from build123d import *

# Parameters (mm, degrees)
BOSS_EXTRUDE1_DEPTH = 2.8
SKETCH2_W           = 22.2
SKETCH2_H           = 5
BOSS_EXTRUDE2_DEPTH = 2.8


with BuildPart() as part:
    # Sketch1 → Boss-Extrude1 (new body)
    with BuildSketch(Plane.XY):
        Polygon((-25, -13.75), (25, -13.75), (25, 13.75), (-25, 13.75), (-25, 23.75), (32.5, 23.75), (32.5, -23.75), (-25, -23.75), align=None)
    extrude(amount=BOSS_EXTRUDE1_DEPTH)

    # Sketch2 → Boss-Extrude2 (add)
    with BuildSketch(Plane(origin=(30, 0, 0), x_dir=(0, 0, -1), z_dir=(1, 0, 0))):
        with BuildLine():
            Line((-2.8, -7.5), (-2.8, 7.5))
            Line((-2.8, 7.5), (-50, 7.5))
            ThreePointArc((-50, 7.5), (-57.5, 0), (-50, -7.5))
            Line((-50, -7.5), (-2.8, -7.5))
        make_face()
        with BuildLine():
            Line((-50, -2.5), (-37.5, -2.5))
            ThreePointArc((-37.5, -2.5), (-35, 0), (-37.5, 2.5))
            Line((-37.5, 2.5), (-50, 2.5))
            ThreePointArc((-50, 2.5), (-52.5, 0), (-50, -2.5))
        make_face(mode=Mode.SUBTRACT)
        with Locations((-18.9, 0)):
            Rectangle(SKETCH2_W, SKETCH2_H, mode=Mode.SUBTRACT)
    extrude(amount=-BOSS_EXTRUDE2_DEPTH)


solid = part.part
Can you work these out from the model? Positions are in its coordinate system, mm. A direction names the side the tool comes from. Round coordinates to 2 decimals unless told otherwise and drop trailing zeros. Loops run counter-clockwise (first coordinate to the right, second up) from the corner with the lowest first, then second, coordinate; pieces in that order, holes last. Notation, with made-up numbers: (36.5, 66.25) - (62.5, 66.25) arc R7 ccw to (62.5, 76.25) - close; hole circle Ø1 at (-10.75, -18.75). An arc over 180 degrees is marked (long way). Answer in a Markdown table with one row per item. Add a question column.
Q1. I want a section at C-C on x = -16. List the corners of the cut face in (y, z) for me.
Q2. We'd pull the mould along Y, two halves only. Please class faces 6 (the flat face through (29, 0, 7.8)), 7 (the flat face through (4, 16, 0)), 8 (the cylindrical face through (29, 0, 35)), 9 (the flat face through (3, 23.75, 1)): pulls with the +Y half, pulls with the -Y half, needs draft (parallel to the pull), parting line crosses it, or undercut.
Q3. I want a section at A-A on y = 0. List the corners of the cut face in (x, z) for me.
Q4. I want a section at B-B on z = 23. List the corners of the cut face in (x, y) for me.
Q5. I want a section at D-D on z = 33.5. List the corners of the cut face in (x, y) for me.
Q6. Which directions (+Z, -Z, +X, -X, +Y, -Y) give clear straight access to the entire face, cutting with the end or side of a thin tool? Please do faces 1 (the flat face through (29, -7.5, 27)), 2 (the flat face through (25, 0, 1)), 3 (the flat face through (30, 0, 31)), 4 (the cylindrical face through (28.6, 0.1, 52.5)), 5 (the flat face through (29, 7.5, 26)).
Q7. I need wall thicknesses on L1, parallel to Y at x = 27.5, z = 40; L2, parallel to Z at x = -7.5, y = -15; L3, parallel to X at y = -3, z = 17.5. Which ranges of each line are inside material? Lowest first, please.
Q8. For pin 1 Ø0.8 at (x, z) = (29, 18) entering from -Y; pin 2 Ø7.5 at (y, z) = (2, 43.5) entering from -X; pin 3 Ø1 at (x, y) = (21, 19) entering from +Z; pin 4 Ø5 at (y, z) = (11.5, 39) entering from +X, each with a flat end and sliding along its axis, tell me the tip position at first contact or that it passes through.
A:
| question | item | result |
|---|---|---|
| 1 | outline | (-23.75, 0) - (-13.75, 0) - (-13.75, 2.8) - (-23.75, 2.8) - close; (13.75, 0) - (23.75, 0) - (23.75, 2.8) - (13.75, 2.8) - close |
| 2 | face 6 | undercut |
| 2 | face 7 | needs draft |
| 2 | face 8 | undercut |
| 2 | face 9 | pulls with the +Y half |
| 3 | outline | (25, 0) - (32.5, 0) - (32.5, 2.8) - (30, 2.8) - (30, 7.8) - (27.2, 7.8) - (27.2, 2.8) - (25, 2.8) - close; (27.2, 30) - (30, 30) - (30, 35) - (27.2, 35) - close; (27.2, 52.5) - (30, 52.5) - (30, 57.5) - (27.2, 57.5) - close |
| 4 | outline | (27.2, -7.5) - (30, -7.5) - (30, -2.5) - (27.2, -2.5) - close; (27.2, 2.5) - (30, 2.5) - (30, 7.5) - (27.2, 7.5) - close |
| 5 | outline | (27.2, -7.5) - (30, -7.5) - (30, 7.5) - (27.2, 7.5) - close |
| 6 | face 1 | +Z, +X, -X, -Y |
| 6 | face 2 | +Z, -Z, -X |
| 6 | face 3 | +Z, +X, +Y, -Y |
| 6 | face 4 | +X, -X |
| 6 | face 5 | +Z, +X, -X, +Y |
| 7 | L1 | -7.5 to -2.5, 2.5 to 7.5 |
| 7 | L2 | 0 to 2.8 |
| 7 | L3 | 27.2 to 30 |
| 8 | pin 1 | y = -7.5 |
| 8 | pin 2 | x = 27.2 |
| 8 | pin 3 | z = 2.8 |
| 8 | pin 4 | through |
